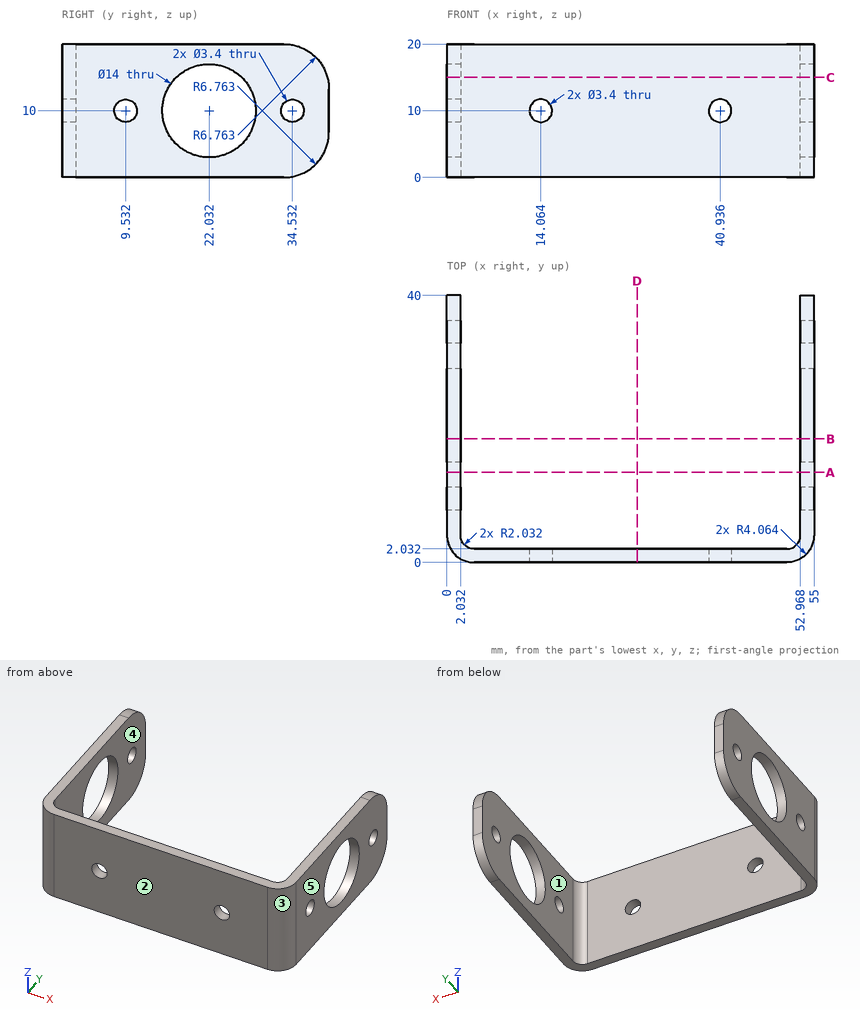
Job drawing, mm, ordinate dimensions from the low corner. One solid piece. A direction names the side the tool comes from. Round coordinates to 2 decimals unless told otherwise and drop trailing zeros. Write each loop counter-clockwise with the first axis right and the second up, starting at its lowest first coordinate (ties: lowest second). Pieces come first, ordered by that corner, then holes.
1) Band-saw the part on D-D, the plane x = 28.5. List the corners of the cut face in (y, z).
2) Band-saw the part on A-A, the plane y = 13.5. List the corners of the cut face in (x, z).
3) Mould opens along X. For the marked faces 1, 2 and 3 say: +X half, -X half, draft (parallel to the pull), parting line (faces both ways), or undercut.
4) Pin check, flat tips, straight feed: pin 1 (3 mm diameter, centred on x = 40.936, z = 10, fed in from +Y); pin 2 (12 mm diameter, centred on x = 16.5, z = 4, fed in from +Y). Stop position of each tip, or through.
5) 3-axis set-ups, long thin cutter, end or side, ignore diameter. For the marked faces 4 and 5: which of +Z, -Z, +X, -X, +Y, -Y reach the whole face in a straight line?
6) Band-saw the part on C-C, the plane z = 15. List the corners of the cut face in (x, y) (1 decimal), and give its area (3 significant figures).
7) Band-saw the part on B-B, the plane y = 18.5. List the corners of the cut face in (x, z).
8) Drill centre lines: probe 1 along X at (y, z) = (13, 9); probe 2 along Y at (x, z) = (1.35, 10); probe 3 along Y at (x, z) = (0.9, 10) (1 decimal). Where is each one in solid material? Low to high.
Ans:
1. outline: (0, 0) - (2.03, 0) - (2.03, 20) - (0, 20) - close
2. outline: (0, 0) - (2.03, 0) - (2.03, 20) - (0, 20) - close; (52.97, 0) - (55, 0) - (55, 20) - (52.97, 20) - close
3. face 1: undercut
3. face 2: draft
3. face 3: +X half
4. pin 1: passes through
4. pin 2: stops at y = 2.03
5. face 4: +Z, -Z, +Y
5. face 5: +Z, -Z, +X, +Y, -Y
6. outline: (0, 4.1) arc R4.1 ccw to (4.1, 0) - (50.9, 0) arc R4.1 ccw to (55, 4.1) - (55, 17.1) - (53, 17.1) - (53, 4.1) arc R2 cw to (50.9, 2) - (4.1, 2) arc R2 cw to (2, 4.1) - (2, 17.1) - (0, 17.1) - close; (0, 26.9) - (2, 26.9) - (2, 39.8) - (0, 39.8) - close; (53, 26.9) - (55, 26.9) - (55, 39.8) - (53, 39.8) - close
6. area: 220 mm2
7. outline: (0, 0) - (2.03, 0) - (2.03, 3.96) - (0, 3.96) - close; (0, 16.04) - (2.03, 16.04) - (2.03, 20) - (0, 20) - close; (52.97, 0) - (55, 0) - (55, 3.96) - (52.97, 3.96) - close; (52.97, 16.04) - (55, 16.04) - (55, 20) - (52.97, 20) - close
8. probe 1: x = 0 to 2.03, 52.97 to 55
8. probe 2: y = 1.04 to 7.83, 11.23 to 15.03, 29.03 to 32.83, 36.23 to 40
8. probe 3: y = 1.5 to 7.8, 11.2 to 15, 29 to 32.8, 36.2 to 40
